from build123d import *

# Parameters (mm, degrees)
EXTRUDE_1_DEPTH     = 39.5
SKETCH_2_R          = 11
EXTRUDE_2_DEPTH     = 2
SKETCH_3_R          = 2.5
EXTRUDE_3_DEPTH     = 22.5
SKETCH_4_W          = 16
SKETCH_4_H          = 5
EXTRUDE_4_DEPTH     = 9.5
SKETCH_5_R          = 1.6
CUT_EXTRUDE_1_DEPTH = 5


with BuildPart() as part:
    # 草图1 → 凸台-拉伸1 (new body)
    with BuildSketch(Plane(origin=(0, 0, 0), x_dir=(1, 0, 0), z_dir=(0, 1, 0))):
        with BuildLine():
            ThreePointArc((0, 7.563061875), (3.37233047, 3.37233047), (7.563061875, 0))
            Line((7.563061875, 0), (34.536938125, 0))
            ThreePointArc((34.536938125, 0), (38.859801315, 3.505457341), (42.3, 7.880432809))
            Line((42.3, 7.880432809), (42.3, 34.219567191))
            ThreePointArc((42.3, 34.219567191), (38.72766953, 38.72766953), (34.219567191, 42.3))
            Line((34.219567191, 42.3), (7.880432809, 42.3))
            ThreePointArc((7.880432809, 42.3), (3.505457341, 38.859801315), (0, 34.536938125))
            Line((0, 34.536938125), (0, 7.563061875))
        make_face()
    extrude(amount=EXTRUDE_1_DEPTH)

    # 草图2 → 凸台-拉伸2 (add)
    with BuildSketch(Plane(origin=(0, 39.5, 0), x_dir=(1, 0, 0), z_dir=(0, 1, 0))):
        with Locations(Location((21.05, 21.05, 0), (0, 0, 270))):
            Circle(SKETCH_2_R)
    extrude(amount=EXTRUDE_2_DEPTH)

    # 草图3 → 凸台-拉伸3 (add)
    with BuildSketch(Plane(origin=(0, 41.5, 0), x_dir=(1, 0, 0), z_dir=(0, 1, 0))):
        with Locations(Location((21.05, 21.05, 0), (0, 0, 90))):
            Circle(SKETCH_3_R)
    extrude(amount=EXTRUDE_3_DEPTH)

    # 草图4 → 凸台-拉伸4 (add)
    with BuildSketch(Plane(origin=(0, 0, 0), x_dir=(1, 0, 0), z_dir=(0, 1, 0))):
        with Locations((21.05, -2.5)):
            Rectangle(SKETCH_4_W, SKETCH_4_H)
    extrude(amount=EXTRUDE_4_DEPTH)

    # 草图5 → 切除-拉伸1 (cut)
    with BuildSketch(Plane(origin=(0, 39.5, 0), x_dir=(1, 0, 0), z_dir=(0, 1, 0))):
        with Locations(Location((5.55, 36.55, 0), (0, 0, 270))):
            Circle(SKETCH_5_R)
        with Locations(Location((36.55, 36.55, 0), (0, 0, 90))):
            Circle(SKETCH_5_R)
        with Locations(Location((36.55, 5.55, 0), (0, 0, 270))):
            Circle(SKETCH_5_R)
        with Locations(Location((5.55, 5.55, 0), (0, 0, 90))):
            Circle(SKETCH_5_R)
    extrude(amount=-CUT_EXTRUDE_1_DEPTH, mode=Mode.SUBTRACT)


solid = part.part
Verification items for the finished model (mm, model axes). A direction names the side the tool comes from. Round coordinates to 2 decimals unless told otherwise and drop trailing zeros. Loops run counter-clockwise (first coordinate to the right, second up) from the corner with the lowest first, then second, coordinate; pieces in that order, holes last. Notation, with made-up numbers: (46.5, 10.25) - (85.5, 10.25) arc R34 cw to (85.5, 45.25) - close; hole circle Ø6 at (17, -32.75). An arc over 180 degrees is marked (long way). Use one line per item in the form item = value.
1. Access from +Z, -Z, +X, -X, +Y, -Y to the whole of each face (thin tool, end or side, straight path). Record for faces 1 (the flat face through (42.3, 19, -21)), 2 (the cylindrical face through (4.2, 37.03, -6.41)), 3 (the flat face through (29.05, 5, 3)).
A:
face_1 = +Z, -Z, +X, +Y, -Y
face_2 = +Y
face_3 = +Z, +X, +Y, -Y
2. Scan lines: probe 1 along X at (y, z) = (37.85, -5.55); probe 2 along X at (y, z) = (36, -5); probe 3 along Y at (x, z) = (12, -3). Record each from-to range of solid material in increasing order.
A:
probe_1 = 1.43 to 3.95, 7.15 to 34.95, 38.15 to 40.67
probe_2 = 1.88 to 4.05, 7.05 to 35.05, 38.05 to 40.22
probe_3 = 0 to 39.5
3. Section check B-B on x = 21.05. Record the cut outline in (y, z).
A:
outline = (0, -42.3) - (39.5, -42.3) - (39.5, -32.05) - (41.5, -32.05) - (41.5, -23.55) - (64, -23.55) - (64, -18.55) - (41.5, -18.55) - (41.5, -10.05) - (39.5, -10.05) - (39.5, 0) - (9.5, 0) - (9.5, 5) - (0, 5) - close
4. Section check A-A on y = 5. Record the cut outline in (x, z), and give its area (3 significant figures).
A:
outline = (0, -34.54) arc R25 ccw to (7.88, -42.3) - (34.22, -42.3) arc R25 ccw to (42.3, -34.22) - (42.3, -7.88) arc R25 ccw to (34.54, 0) - (29.05, 0) - (29.05, 5) - (13.05, 5) - (13.05, 0) - (7.56, 0) arc R25 ccw to (0, -7.56) - close
area = 1,770 mm²
5. Section check D-D on z = -14.5. Record the cut outline in (x, y).
A:
outline = (0, 0) - (42.3, 0) - (42.3, 39.5) - (29.89, 39.5) - (29.89, 41.5) - (12.21, 41.5) - (12.21, 39.5) - (0, 39.5) - close
6. Gauge pin test, flat ends, axial feed: pin 1 Ø2.5 at (x, z) = (5.55, -36.55) entering from -Y; pin 2 Ø10 at (x, y) = (18, 54.5) entering from -Z; pin 3 Ø2.5 at (x, z) = (5.55, -5.55) entering from +Y; pin 4 Ø5.5 at (x, z) = (20, 3.5) entering from +Y. Record the tip position at first contact, or that the pin passes through.
A:
pin_1 = 0
pin_2 = -23.55
pin_3 = 34.5
pin_4 = 9.5
7. Draft check along Z on faces 4 (the flat face through (6, 34.5, -37)), 5 (the cylindrical face through (38.805, 19.474, -3.45)), 6 (the flat face through (21, 9.5, 2)), 7 (the cylindrical face through (5.62, 37.03, -38.15)). Enter one of: pulls with the +Z half, pulls with the -Z half, needs draft (parallel to the pull), parting line crosses it, or undercut.
A:
face_4 = undercut
face_5 = pulls with the +Z half
face_6 = needs draft
face_7 = undercut
8. Section check C-C on z = -21.05. Record the cut outline in (x, y).
A:
outline = (0, 0) - (42.3, 0) - (42.3, 39.5) - (32.05, 39.5) - (32.05, 41.5) - (23.55, 41.5) - (23.55, 64) - (18.55, 64) - (18.55, 41.5) - (10.05, 41.5) - (10.05, 39.5) - (0, 39.5) - close
